Check sheet for the modelled part. Datum: model origin and axes. Units: mm. Face numbers are marked on the shaded views. Coordinates: 2 decimals unless noted, no trailing zeros. Loops run counter-clockwise (first coordinate to the right, second up) from the corner with the lowest first, then second, coordinate; pieces in that order, holes last.
```python
from build123d import *

# Parameters (mm, degrees)
SKETCH_1_R               = 9.25
SKETCH_1_R_2             = 2.5
EXTRUDE_1_DEPTH          = 7.5
SKETCH_3_R               = 1.75
CUT_EXTRUDE_1_DEPTH      = 16.5
CUT_EXTRUDE_1_DEPTH_BACK = 16.5
CHAMFER_1_SIZE           = 1
CHAMFER_2_SIZE           = 1


with BuildPart() as part:
    # ｽｹｯﾁ1 → ﾎﾞｽ - 押し出し1 (new body, symmetric)
    with BuildSketch(Plane.XY):
        with BuildLine():
            Line((2.683281573, 19.807546152), (12.183281573, 15.057546152))
            ThreePointArc((12.183281573, 15.057546152), (14.60390485, 12.845369678), (15.5, 9.690983006))
            Line((15.5, 9.690983006), (15.5, -9.5))
            ThreePointArc((15.5, -9.5), (13.742640687, -13.742640687), (9.5, -15.5))
            Line((9.5, -15.5), (-9.5, -15.5))
            ThreePointArc((-9.5, -15.5), (-13.742640687, -13.742640687), (-15.5, -9.5))
            Line((-15.5, -9.5), (-15.5, 9.690983006))
            ThreePointArc((-15.5, 9.690983006), (-14.60390485, 12.845369678), (-12.183281573, 15.057546152))
            Line((-12.183281573, 15.057546152), (-2.683281573, 19.807546152))
            ThreePointArc((-2.683281573, 19.807546152), (0, 20.440983006), (2.683281573, 19.807546152))
        make_face()
        Circle(SKETCH_1_R, mode=Mode.SUBTRACT)
        with Locations((-10, -10)):
            Circle(SKETCH_1_R_2, mode=Mode.SUBTRACT)
        with Locations((-10, 10)):
            Circle(SKETCH_1_R_2, mode=Mode.SUBTRACT)
        with Locations((10, 10)):
            Circle(SKETCH_1_R_2, mode=Mode.SUBTRACT)
        with Locations((10, -10)):
            Circle(SKETCH_1_R_2, mode=Mode.SUBTRACT)
        with Locations((0, 15)):
            Circle(SKETCH_1_R_2, mode=Mode.SUBTRACT)
    extrude(amount=EXTRUDE_1_DEPTH, both=True)

    # ｽｹｯﾁ3 → ｶｯﾄ - 押し出し1 (cut, two sides)
    with BuildSketch(Plane(origin=(0, 0, 0), x_dir=(0, 0, -1), z_dir=(1, 0, 0))) as cut_extrude_1_sk:
        Circle(SKETCH_3_R)
    extrude(amount=CUT_EXTRUDE_1_DEPTH, mode=Mode.SUBTRACT)
    extrude(cut_extrude_1_sk.sketch, amount=-CUT_EXTRUDE_1_DEPTH_BACK, mode=Mode.SUBTRACT)

    # 面取り1
    chamfer_1_edges = [part.edges().sort_by_distance(p)[0] for p in [
        (-12.5, -10, -7.5),
        (-12.5, -10, 7.5),
        (-12.5, 10, -7.5),
        (-12.5, 10, 7.5),
        (7.5, 10, -7.5),
        (7.5, 10, 7.5),
        (7.5, -10, -7.5),
        (7.5, -10, 7.5),
        (-2.5, 15, -7.5),
        (-2.5, 15, 7.5),
    ]]
    chamfer(chamfer_1_edges, length=CHAMFER_1_SIZE)

    # 面取り2
    chamfer_2_edges = [part.edges().sort_by_distance(p)[0] for p in [
        (-15.5, 0.095491503, -7.5),
        (-14.60390485, 12.845369678, -7.5),
        (-7.433281573, 17.432546152, -7.5),
        (0, 20.440983006, -7.5),
        (7.433281573, 17.432546152, -7.5),
        (14.60390485, 12.845369678, -7.5),
        (15.5, 0.095491503, -7.5),
        (13.742640687, -13.742640687, 7.5),
        (13.742640687, -13.742640687, -7.5),
        (0, -15.5, -7.5),
        (-13.742640687, -13.742640687, -7.5),
        (15.5, 0.095491503, 7.5),
        (14.60390485, 12.845369678, 7.5),
        (7.433281573, 17.432546152, 7.5),
        (0, 20.440983006, 7.5),
        (-7.433281573, 17.432546152, 7.5),
        (-14.60390485, 12.845369678, 7.5),
        (-15.5, 0.095491503, 7.5),
        (-13.742640687, -13.742640687, 7.5),
        (0, -15.5, 7.5),
    ]]
    chamfer(chamfer_2_edges, length=CHAMFER_2_SIZE)


solid = part.part
```
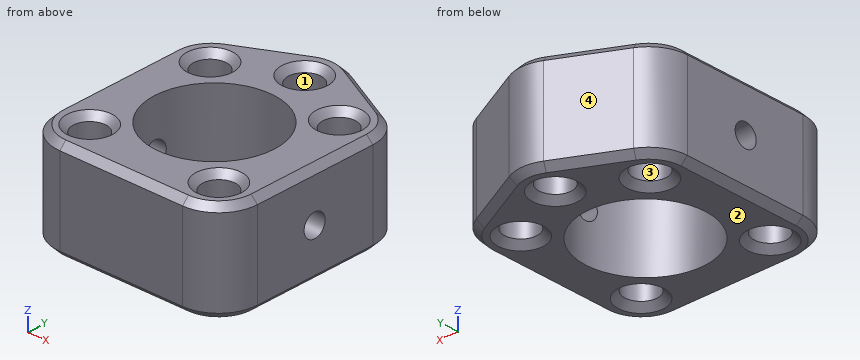
1) Scan lines: line 1 (Y direction, x = 0, z = 1.25); line 2 (Y direction, x = -10, z = 2); line 3 (Y direction, x = 5, z = 4.75). Record each from-to range of solid material in increasing order.
Answer sheet:
line 1: y = -15.5 to -9.25, 9.25 to 12.5, 17.5 to 20.44
line 2: y = -15.48 to -12.5, -7.5 to 7.5, 12.5 to 16.15
line 3: y = -15.5 to -7.78, 7.78 to 18.65
2) Section check C-C on z = -1.25. Enter the section's corners in (x, y), plus the area to 3 significant figures.
Answer sheet:
outline: (-15.5, -9.5) arc R6 ccw to (-9.5, -15.5) - (9.5, -15.5) arc R6 ccw to (15.5, -9.5) - (15.5, -1.22) - (9.17, -1.22) arc R9.25 cw to (-9.17, -1.22) - (-15.5, -1.22) - close; (-15.5, 1.22) - (-9.17, 1.22) arc R9.25 cw to (9.17, 1.22) - (15.5, 1.22) - (15.5, 9.69) arc R6 ccw to (12.18, 15.06) - (2.68, 19.81) arc R6 ccw to (-2.68, 19.81) - (-12.18, 15.06) arc R6 ccw to (-15.5, 9.69) - close; hole circle Ø5 at (-10, -10); hole circle Ø5 at (-10, 10); hole circle Ø5 at (0, 15); hole circle Ø5 at (10, -10); hole circle Ø5 at (10, 10)
area: 597 mm2
3) Depth check by flat-ended pin: pin 1 (6 mm diameter, centred on y = 13, z = 1, fed in from -X); pin 2 (2 mm diameter, centred on x = 8.5, y = -1, fed in from +Z); pin 3 (6 mm diameter, centred on x = -10, y = -10, fed in from -Z); pin 4 (4 mm diameter, centred on y = 15.5, z = 3.5, fed in from +X). Enter the tip coordinate at first touch or a pass-through.
Answer sheet:
pin 1: stops at x = -15.49
pin 2: stops at z = 7.5
pin 3: stops at z = -7
pin 4: stops at x = 14.14
4) Section check B-B on z = -5.25. Enter the section's corners in (x, y), plus the area to 3 significant figures.
Answer sheet:
outline: (-15.5, -9.5) arc R6 ccw to (-9.5, -15.5) - (9.5, -15.5) arc R6 ccw to (15.5, -9.5) - (15.5, 9.69) arc R6 ccw to (12.18, 15.06) - (2.68, 19.81) arc R6 ccw to (-2.68, 19.81) - (-12.18, 15.06) arc R6 ccw to (-15.5, 9.69) - close; hole circle Ø5 at (-10, -10); hole circle Ø5 at (-10, 10); hole circle Ø18.5 at (0, 0); hole circle Ø5 at (0, 15); hole circle Ø5 at (10, -10); hole circle Ø5 at (10, 10)
area: 628 mm2
5) Section check A-A on y = 0. Enter the section's corners in (x, z).
Answer sheet:
outline: (-15.5, -6.5) - (-14.5, -7.5) - (-9.25, -7.5) - (-9.25, -1.75) - (-15.5, -1.75) - close; (-15.5, 1.75) - (-9.25, 1.75) - (-9.25, 7.5) - (-14.5, 7.5) - (-15.5, 6.5) - close; (9.25, -7.5) - (14.5, -7.5) - (15.5, -6.5) - (15.5, -1.75) - (9.25, -1.75) - close; (9.25, 1.75) - (15.5, 1.75) - (15.5, 6.5) - (14.5, 7.5) - (9.25, 7.5) - close
6) Mould release check, pull along X, two halves, no side actions. Record for the marked faces 1, 2, 3 and 4: +X half, -X half, draft (parallel to the pull), parting line (faces both ways), or undercut.
Answer sheet:
face 1: undercut
face 2: draft
face 3: undercut
face 4: -X half
7) Section check D-D on x = 11. Give the number of separate pieces and of enclosed holes in the cut face, plus the area to 3 significant figures.
Answer sheet:
separate pieces: 3
enclosed holes: 1
area: 311 mm2
